Can you work these out from the model? Positions are in its coordinate system, mm. A direction names the side the tool comes from. Give positions to 0.01 mm unless a question says otherwise; leave off trailing zeros. Loops run counter-clockwise (first coordinate to the right, second up) from the corner with the lowest first, then second, coordinate; pieces in that order, holes last.
from build123d import *

# Parameters (mm, degrees)
F0_R     = 50
F1_DEPTH = 5
F2_R     = 10
F3_DEPTH = 100
F4_R     = 9.2
F5_DEPTH = 95
F6_SIZE  = 1


with BuildPart() as f1:
    # F0 (on Top) → F1 (new body)
    with BuildSketch(Plane.XY):
        Circle(F0_R)
    extrude(amount=F1_DEPTH)

    # F2 (on face) → F3 (join)
    with BuildSketch(Plane.XY.offset(5)):
        Circle(F2_R)
    extrude(amount=F3_DEPTH)

    # F4 (on face) → F5 (cut, through all)
    with BuildSketch(Plane.XY.offset(105)):
        Circle(F4_R)
    extrude(amount=-F5_DEPTH, mode=Mode.SUBTRACT)

    # F6
    f6_edges = [f1.edges().sort_by_distance(p)[0] for p in [
        (-50, 0, 5),
        (-50, 0, 0),
    ]]
    chamfer(f6_edges, length=F6_SIZE)

    # F7 (on Front) → F8 (revolve)
    with BuildSketch(Plane.XZ):
        with BuildLine():
            Line((9.2, 105), (10, 105))
            ThreePointArc((10, 105), (7.0710678119, 112.0710678119), (0, 115))
            Line((0, 115), (0, 114.2))
            ThreePointArc((0, 114.2), (6.5053823869, 111.5053823869), (9.2, 105))
        make_face()
    revolve(axis=Axis((0, 0, 109.6), (0, 0, 1)))


solid = f1.part
(1) Suppose I cut it at C-C on z = 8.5. List the corners of the cut face in (x, y) for me.
Returned:
outline: circle Ø20 at (0, 0)
(2) Suppose I cut it at A-A on y = 0. List the corners of the cut face in (x, z) for me.
Returned:
outline: (-50, 1) - (-49, 0) - (49, 0) - (50, 1) - (50, 4) - (49, 5) - (10, 5) - (10, 105) arc R10 ccw to (-10, 105) - (-10, 5) - (-49, 5) - (-50, 4) - close; hole (-9.2, 10) - (9.2, 10) - (9.2, 105) arc R9.2 ccw to (-9.2, 105) - close
(3) Which directions (+Z, -Z, +X, -X, +Y, -Y) give clear straight access to the entire face, cutting with the end or side of a thin tool? Please do faces 1 (the flat face through (0, 0, 10)), 2 (the flat face through (-1, 1, 0)), 3 (the cylindrical face through (-2.17, -9.76, 54.3)).
Returned:
face 1: none
face 2: -Z, +X, -X, +Y, -Y
face 3: +Z
(4) Please list where these lines run through material, in increasing order: probe 1 along Y at (x, z) = (0, 51); probe 2 along Z at (x, y) = (20, 32.5); probe 3 along Y at (x, z) = (2, 94.5).
Returned:
probe 1: y = -10 to -9.2, 9.2 to 10
probe 2: z = 0 to 5
probe 3: y = -9.8 to -8.98, 8.98 to 9.8
(5) Thinking about a two-plate mould opening in Y: for faces 4 (the cylindrical face through (-7.3, -5.6, 58.2)), 5 (the flat face through (10.2, 0.7, 5)), 6 (the cylindrical face through (47.69, 15.02, 2.48)), which applies, pulls with the +Y half, pulls with the -Y half, needs draft (parallel to the pull), parting line crosses it, or undercut?
Returned:
face 4: undercut
face 5: needs draft
face 6: parting line crosses it
(6) Suppose I cut it at D-D on z = 87. List the corners of the cut face in (x, y) for me, plus the area to 3 significant figures.
Returned:
outline: circle Ø20 at (0, 0); hole circle Ø18.4 at (0, 0)
area: 48.3 mm2
(7) Will this pin go through, and if not, where does the flat tip stop? P1, Ø8, axis at x = -6, y = -20.5, coming from the +Z side.
Returned:
P1: stops at z = 5
